Here's how the part is built. I have some questions about the finished solid (model axes, mm). Face numbers are marked on the shaded views. A direction names the side the tool comes from. Give positions to 0.01 mm unless a question says otherwise; leave off trailing zeros. Loops run counter-clockwise (first coordinate to the right, second up) from the corner with the lowest first, then second, coordinate; pieces in that order, holes last. Notation, with made-up numbers: (-6, 80.25) - (-2, 80.25) arc R7 ccw to (-2, 87.25) - close; hole circle Ø1 at (42, -16). An arc over 180 degrees is marked (long way). Return JSON: item names as keys, results as strings. Group by question number.
(1) For P1, Ø5, axis at y = -9, z = 10, coming from the +X side; P2, Ø5, axis at x = 9.5, z = 9.5, coming from the -Y side; P3, Ø3, axis at y = -11, z = 8.5, coming from the -X side; P4, Ø3, axis at x = 0, y = -8.3, coming from the +Z side, each with a flat end and sliding along its axis, tell me the tip position at first contact or that it passes through.
(2) On a 3-axis mill with a long thin cutter (end or side, diameter ignored), from which of +Z, -Z, +X, -X, +Y, -Y can I reach the whole of each face in a straight line? I mean the marked faces 1, 2, 3, 4 and 5. Say none if no direction works.
(3) If we section it at A-A (y = -12): Please give me the cut outline in (x, z).
(4) I need wall thicknesses on probe 1 along Y at (x, z) = (20, 2.35); probe 2 along X at (y, z) = (-6.3, 10); probe 3 along X at (y, z) = (-11.5, 11). Which ranges of each line are inside material? Lowest first, please. Write a range as [from, to].
(5) If we section it at C-C (x = 0): Please give me the cut outline in (y, z), then the cut area to 3 significant figures.
(6) If we section it at B-B (y = -6.75): Please give me the cut outline in (x, z).
(7) If we section it at D-D (z = 10): Please give me the cut outline in (x, y).
(8) If we mould it in two halves opening along X, with no side actions, what happens to the marked faces 6, 7 and 8? For each: released by +X, released by -X, zero draft, split by the parting line, or undercut.
```python
from build123d import *

# Parameters (mm, degrees)
SKETCH1_W               = 30
SKETCH1_H               = 10
SKETCH1_R               = 2
BOSS_EXTRUDE1_DEPTH     = 3
SKETCH2_W               = 10
SKETCH2_H               = 10
BOSS_EXTRUDE2_DEPTH     = 15
CUT_EXTRUDE1_START      = -10
SKETCH3_R               = 2
CUT_EXTRUDE1_DEPTH      = 5
CUT_EXTRUDE2_DEPTH      = 33.388269481
CUT_EXTRUDE2_DEPTH_BACK = 33.388269481
SKETCH3_2_R             = 2


with BuildPart() as part:
    # Sketch1 → Boss-Extrude1 (new body)
    with BuildSketch(Plane.XY):
        with Locations((10, -8.3)):
            Rectangle(SKETCH1_W, SKETCH1_H)
        with Locations((20, -8.3)):
            Circle(SKETCH1_R, mode=Mode.SUBTRACT)
        with Locations(Location((0, -8.3, 0), (0, 0, 180))):
            Circle(SKETCH1_R, mode=Mode.SUBTRACT)
    extrude(amount=BOSS_EXTRUDE1_DEPTH)

    # Sketch2 → Boss-Extrude2 (add)
    with BuildSketch(Plane.XY.offset(3)):
        with Locations((10, -8.3)):
            Rectangle(SKETCH2_W, SKETCH2_H)
    extrude(amount=BOSS_EXTRUDE2_DEPTH)

    # Sketch3 → Cut-Extrude1 (cut)
    with BuildSketch(Plane(origin=(0, -3.3, 0), x_dir=(1, 0, 0), z_dir=(0, 1, 0)).offset(CUT_EXTRUDE1_START)):
        Polygon((10, -6.07401817), (6.6, -8.037009085), (6.6, -11.962990915), (10, -13.92598183), (13.4, -11.962990915), (13.4, -8.037009085), align=None)
        with Locations(Location((10, -10, 0), (0, 0, 270))):
            Circle(SKETCH3_R, mode=Mode.SUBTRACT)
    extrude(amount=CUT_EXTRUDE1_DEPTH, mode=Mode.SUBTRACT)

    # Sketch3<2> → Cut-Extrude2 (cut, two sides: drawn at the far end of the back side and taken through both)
    with BuildSketch(Plane(origin=(0, -3.3, 0), x_dir=(1, 0, 0), z_dir=(0, 1, 0)).offset(-CUT_EXTRUDE2_DEPTH_BACK)):
        with Locations(Location((10, -10, 0), (0, 0, 270))):
            Circle(SKETCH3_2_R)
    extrude(amount=CUT_EXTRUDE2_DEPTH + CUT_EXTRUDE2_DEPTH_BACK, mode=Mode.SUBTRACT)


solid = part.part
```
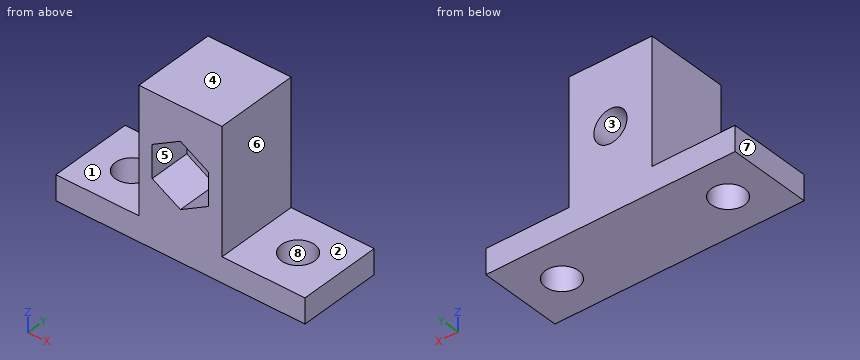
Values:
{
 "1": {"P1": "x = 15", "P2": "y = -8.3", "P3": "x = 5", "P4": "through"},
 "2": {"face 1": "+Z, -X, +Y, -Y", "face 2": "+Z, +X, +Y, -Y", "face 3": "+Y, -Y", "face 4": "+Z, +X, -X, +Y, -Y", "face 5": "-Y"},
 "3": {"outline": "(-5, 0) - (25, 0) - (25, 3) - (15, 3) - (15, 18) - (5, 18) - (5, 3) - (-5, 3) - close; hole (6.6, 8.04) - (10, 6.07) - (13.4, 8.04) - (13.4, 11.96) - (10, 13.93) - (6.6, 11.96) - close"},
 "4": {"probe 1": "[-13.3, -10.3], [-6.3, -3.3]", "probe 2": "[5, 8], [12, 15]", "probe 3": "[5, 6.6], [13.4, 15]"},
 "5": {"outline": "(-13.3, 0) - (-10.3, 0) - (-10.3, 3) - (-13.3, 3) - close; (-6.3, 0) - (-3.3, 0) - (-3.3, 3) - (-6.3, 3) - close", "area": "18.0 mm2"},
 "6": {"outline": "(-5, 0) - (-1.26, 0) - (-1.26, 3) - (-5, 3) - close; (1.26, 0) - (18.74, 0) - (18.74, 3) - (15, 3) - (15, 18) - (5, 18) - (5, 3) - (1.26, 3) - close; (21.26, 0) - (25, 0) - (25, 3) - (21.26, 3) - close; hole circle Ø4 at (10, 10)"},
 "7": {"outline": "(5, -13.3) - (6.6, -13.3) - (6.6, -8.3) - (8, -8.3) - (8, -3.3) - (5, -3.3) - close; (12, -8.3) - (13.4, -8.3) - (13.4, -13.3) - (15, -13.3) - (15, -3.3) - (12, -3.3) - close"},
 "8": {"face 6": "released by +X", "face 7": "released by -X", "face 8": "undercut"}
}
